Check sheet for the modelled part. Datum: model origin and axes. Units: mm. Face numbers are marked on the shaded views. A direction names the side the tool comes from. Round coordinates to 2 decimals unless told otherwise and drop trailing zeros. Write each loop counter-clockwise with the first axis right and the second up, starting at its lowest first coordinate (ties: lowest second). Pieces come first, ordered by that corner, then holes.
Item 1: Material ranges on line 1 (Z direction, x = 51, y = 0) (3 decimals); line 2 (Z direction, x = 75, y = 0) (3 decimals); line 3 (X direction, y = -6, z = 23), recorded low to high.
Item 2: Cross-section at A-A on z = 0. Enter the section's corners in (x, y) (3 decimals).
Item 3: Cross-section at D-D on y = -7.5. Enter the section's corners in (x, z) (3 decimals).
Item 4: Cross-section at C-C on y = 15.5. Enter the section's corners in (x, z) (3 decimals), plus the area to 3 significant figures.
Item 5: Go/stop test with flat-tipped pins: pin 1 Ø1.5 at (x, y) = (70, -2.5) entering from +Z; pin 2 Ø2 at (x, z) = (118.5, 1) entering from +Y; pin 3 Ø6 at (x, y) = (73.5, 11) entering from -Z; pin 4 Ø17 at (y, z) = (0, 0) entering from +X. Record where each tip stops, or that it passes through.
Item 6: Release check for a two-part mould opening along Z. For the marked faces 3, 4 and 5 record: +Z half, -Z half, draft (parallel to the pull), parting line (faces both ways), or undercut.
Item 7: Tool access check on the marked faces 1 and 2. Record the directions out of +Z, -Z, +X, -X, +Y, -Y that give a thin tool (end or side, any length) a straight path to the whole face; none if there is none.
from build123d import *

# Parameters (mm, degrees)
CUT_EXTRUDE1_DEPTH = 6.35
SKETCH3_R          = 9.525
CUT_EXTRUDE2_DEPTH = 160.668095298


with BuildPart() as part:
    # Sketch1 → Revolve1 (revolve)
    with BuildSketch(Plane.XY):
        Polygon((155.575, 0), (0, 0), (0, 25.4), (12.7, 25.4), (12.7, 18.923), (155.575, 18.923), align=None)
    revolve(axis=Axis((155.575, 0, 0), (-1, 0, 0)))

    # Sketch2 → Cut-Extrude1 (cut)
    with BuildSketch(Plane.XY.offset(18.923)):
        with BuildLine():
            Line((74.6125, 0), (155.575, 0))
            Line((155.575, 0), (155.575, 4.7625))
            Line((155.575, 4.7625), (79.375, 4.7625))
            ThreePointArc((79.375, 4.7625), (76.007403955, 3.367596045), (74.6125, 0))
        make_face()
        with BuildLine():
            Line((155.575, -4.7625), (155.575, 0))
            Line((155.575, 0), (74.6125, 0))
            ThreePointArc((74.6125, 0), (76.007403955, -3.367596045), (79.375, -4.7625))
            Line((79.375, -4.7625), (155.575, -4.7625))
        make_face()
    extrude(amount=-CUT_EXTRUDE1_DEPTH, mode=Mode.SUBTRACT)

    # Sketch3 → Cut-Extrude2 (cut, through all)
    with BuildSketch(Plane.ZY):
        with Locations(Location((0, 0, 0), (0, 0, 270))):
            Circle(SKETCH3_R)
    extrude(amount=-CUT_EXTRUDE2_DEPTH, mode=Mode.SUBTRACT)


solid = part.part
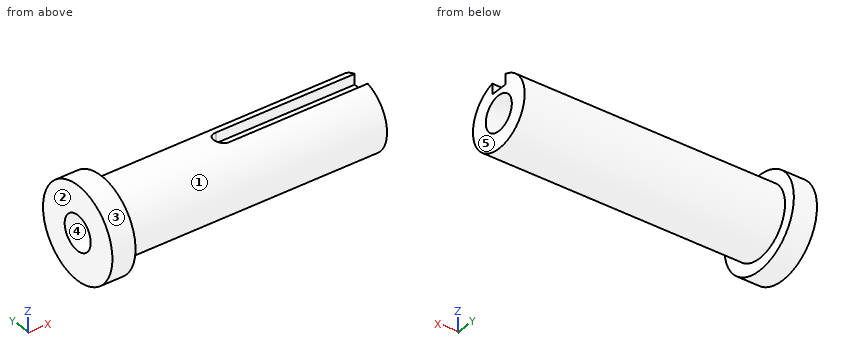
Response values:
1. line 1: z = -18.923 to -9.525, 9.525 to 18.923
1. line 2: z = -18.923 to -9.525, 9.525 to 12.573
1. line 3: x = 0 to 12.7
2. outline: (0, -25.4) - (12.7, -25.4) - (12.7, -18.923) - (155.575, -18.923) - (155.575, -9.525) - (0, -9.525) - close; (0, 9.525) - (155.575, 9.525) - (155.575, 18.923) - (12.7, 18.923) - (12.7, 25.4) - (0, 25.4) - close
3. outline: (0, -24.267) - (12.7, -24.267) - (12.7, -17.373) - (155.575, -17.373) - (155.575, -5.872) - (0, -5.872) - close; (0, 5.872) - (155.575, 5.872) - (155.575, 17.373) - (12.7, 17.373) - (12.7, 24.267) - (0, 24.267) - close
4. outline: (0, -20.122) - (12.7, -20.122) - (12.7, -10.855) - (155.575, -10.855) - (155.575, 10.855) - (12.7, 10.855) - (12.7, 20.122) - (0, 20.122) - close
4. area: 3,610 mm2
5. pin 1: stops at z = 18.84
5. pin 2: stops at y = 18.92
5. pin 3: stops at z = -17.15
5. pin 4: passes through
6. face 3: parting line
6. face 4: undercut
6. face 5: draft
7. face 1: +X
7. face 2: +Z, -Z, -X, +Y, -Y
